The listing builds one solid part. Answer for the finished solid, in the listing's coordinates (mm). A direction names the side the tool comes from. Give positions to 0.01 mm unless a question says otherwise; leave off trailing zeros. Order: outer loops, then holes, each group sorted by start corner. A loop starts at its lowest first (then second) coordinate and runs counter-clockwise, first axis right, second up. Notation, with made-up numbers: (-30.5, 64.25) -> (-22.5, 64.25) arc R9 cw to (-22.5, 77.25) -> close; hole circle Ø7 at (-28, -8.5). An arc over 180 degrees is marked (long way). Answer as a JSON object with one key per item and string values. Group by question number.
```python
from build123d import *

# Parameters (mm, degrees)
F1_DEPTH = 6.35
F3_D     = 3.175
F3_DEPTH = 12.7
F3_TIP   = 0.9538662327


with BuildPart() as f1:
    # F0 (on Right) → F1 (new body)
    with BuildSketch(Plane.YZ):
        with BuildLine():
            Line((0, 50.8), (0, 0))
            Line((0, 0), (25.4, 0))
            Line((25.4, 0), (25.4, 50.8))
            ThreePointArc((25.4, 50.8), (12.7, 38.1), (0, 50.8))
        make_face()
        with BuildLine():
            Line((9.525, 50.8), (0, 50.8))
            ThreePointArc((0, 50.8), (12.7, 38.1), (25.4, 50.8))
            Line((25.4, 50.8), (15.875, 50.8))
            ThreePointArc((15.875, 50.8), (12.7, 47.625), (9.525, 50.8))
        make_face()
        with BuildLine():
            ThreePointArc((25.4, 50.8), (12.7, 63.5), (0, 50.8))
            Line((0, 50.8), (9.525, 50.8))
            ThreePointArc((9.525, 50.8), (12.7, 53.975), (15.875, 50.8))
            Line((15.875, 50.8), (25.4, 50.8))
        make_face()
    extrude(amount=F1_DEPTH)

    # F3
    with Locations(Plane(origin=(0, 0, 0), x_dir=(1, 0, 0), z_dir=(0, 0, -1))):
        with Locations((3.175, -3.175), (3.175, -22.225)):
            Hole(F3_D / 2, depth=F3_DEPTH)
            with Locations((0, 0, -(F3_DEPTH + F3_TIP / 2))):  # 118° drill point
                Cone(0, F3_D / 2, F3_TIP, mode=Mode.SUBTRACT)


solid = f1.part
```
(1) A cutting plane is placed at D-D (y = 7.75). Determine the outline of the cut face in (x, z).
(2) Flat-ended cylindrical pins translate along their axes: pin 1 Ø4 at (y, z) = (12.7, 50.8) entering from -X; pin 2 Ø2 at (x, y) = (2.5, 14.5) entering from -Z; pin 3 Ø1.9 at (x, y) = (3.175, 3.175) entering from -Z; pin 4 Ø2 at (x, y) = (4, 22) entering from +Z. Find the tip coordinate at first contact, or state that the pin passes through.
(3) For a pull along X with two mould halves and no side action, classify faces 1 (the flat face through (3, 13, 0)), 2 (the cylindrical face through (3.519, 4.725, 6.439)), 3 (the flat face through (0, 13, 32)) as +X half, -X half, draft (parallel to the pull), parting line (faces both ways), or undercut.
(4) A cutting plane is placed at B-B (z = 51.5). Determine the outline of the cut face in (x, y), and give its area (3 significant figures).
(5) A cutting plane is placed at A-A (y = 12.7). Determine the outline of the cut face in (x, z) (3 decimals).
(6) Find the intervals of material crossed by line 1 along Z through (x, y) = (4.5, 12.7) (3 decimals); line 2 along Y through (x, z) = (2, 6); line 3 along Z through (x, y) = (4.75, 14), in increasing order. Write a range as [from, to].
(7) A cutting plane is placed at C-C (x = 1). Determine the outline of the cut face in (y, z) (3 decimals), and give its area (3 significant figures).
(8) Which of the six approach directions +Z, -Z, +X, -X, +Y, -Y give full straight-line access (tool end or side, diameter ignored) to faces 4 (the cylindrical face through (3.13, 13.11, 53.95)), 5 (the cylindrical face through (3.38, 20.65, 6.44))?
Check sheet entries:
{
 "1": {"outline": "(0, 0) -> (6.35, 0) -> (6.35, 62.5) -> (0, 62.5) -> close"},
 "2": {"pin 1": "passes through", "pin 2": "stops at z = 0", "pin 3": "stops at z = 13.08", "pin 4": "stops at z = 60.41"},
 "3": {"face 1": "draft", "face 2": "undercut", "face 3": "-X half"},
 "4": {"outline": "(0, 0.02) -> (6.35, 0.02) -> (6.35, 9.6) -> (0, 9.6) -> close; (0, 15.8) -> (6.35, 15.8) -> (6.35, 25.38) -> (0, 25.38) -> close", "area": "122 mm2"},
 "5": {"outline": "(0, 0) -> (6.35, 0) -> (6.35, 47.625) -> (0, 47.625) -> close; (0, 53.975) -> (6.35, 53.975) -> (6.35, 63.5) -> (0, 63.5) -> close"},
 "6": {"line 1": "z = [0, 47.625], [53.975, 63.5]", "line 2": "y = [0, 2.11], [4.24, 21.16], [23.29, 25.4]", "line 3": "z = [0, 47.9], [53.7, 63.43]"},
 "7": {"outline": "(0, 0) -> (25.4, 0) -> (25.4, 50.8) arc R12.7 ccw to (0, 50.8) -> close; hole circle Ø6.35 at (12.7, 50.8)", "area": "1,510 mm2"},
 "8": {"face 4": "+X, -X", "face 5": "-Z"}
}
